Check sheet for the modelled part. Datum: model origin and axes. Units: mm. Face numbers are marked on the shaded views. A direction names the side the tool comes from. Coordinates: 2 decimals unless noted, no trailing zeros. Loops run counter-clockwise (first coordinate to the right, second up) from the corner with the lowest first, then second, coordinate; pieces in that order, holes last.
```python
from build123d import *
from build123d import SkipClean  # not in build123d's __all__

# Parameters (mm, degrees)
F0_R     = 37.5
F0_R_2   = 4.75
F1_DEPTH = 4
F2_DEPTH = 12


with BuildPart() as f1:
    # F0 (on Top) → F1 (new body)
    with BuildSketch(Plane.XY):
        Circle(F0_R)
        with BuildLine():
            ThreePointArc((3.5, 24.753787589), (18.8745860882, 16.3935963108), (25, 0))
            ThreePointArc((25, 0), (24.5426691937, -4.7599778204), (23.1874088919, -9.3458048812))
            ThreePointArc((23.1874088919, -9.3458048812), (21.6506350946, -12.5), (19.6874088919, -15.4079827077))
            ThreePointArc((19.6874088919, -15.4079827077), (0, -25), (-19.6874088919, -15.4079827077))
            ThreePointArc((-19.6874088919, -15.4079827077), (-21.6506350946, -12.5), (-23.1874088919, -9.3458048812))
            ThreePointArc((-23.1874088919, -9.3458048812), (-21.6506350946, 12.5), (-3.5, 24.753787589))
            ThreePointArc((-3.5, 24.753787589), (0, 25), (3.5, 24.753787589))
        make_face(mode=Mode.SUBTRACT)
        with BuildLine():
            Line((3.5, 21.719806629), (3.5, 24.753787589))
            ThreePointArc((3.5, 24.753787589), (0, 25), (-3.5, 24.753787589))
            Line((-3.5, 24.753787589), (-3.5, 21.719806629))
            ThreePointArc((-3.5, 21.719806629), (0, 22), (3.5, 21.719806629))
        make_face()
        with BuildLine():
            Line((3.5, 9.3674969976), (3.5, 21.719806629))
            ThreePointArc((3.5, 21.719806629), (0, 22), (-3.5, 21.719806629))
            Line((-3.5, 21.719806629), (-3.5, 9.3674969976))
            ThreePointArc((-3.5, 9.3674969976), (0, 10), (3.5, 9.3674969976))
        make_face()
        with BuildLine():
            ThreePointArc((17.059904306, -13.8909922277), (19.0525588833, -11), (20.559904306, -7.8288144012))
            Line((20.559904306, -7.8288144012), (9.8624903698, -1.6526595856))
            ThreePointArc((9.8624903698, -1.6526595856), (8.6602540378, -5), (6.3624903698, -7.714837412))
            Line((6.3624903698, -7.714837412), (17.059904306, -13.8909922277))
        make_face()
        with BuildLine():
            ThreePointArc((19.6874088919, -15.4079827077), (21.6506350946, -12.5), (23.1874088919, -9.3458048812))
            Line((23.1874088919, -9.3458048812), (20.559904306, -7.8288144012))
            ThreePointArc((20.559904306, -7.8288144012), (19.0525588833, -11), (17.059904306, -13.8909922277))
            Line((17.059904306, -13.8909922277), (19.6874088919, -15.4079827077))
        make_face()
        with BuildLine():
            Line((-9.8624903698, -1.6526595856), (-20.559904306, -7.8288144012))
            ThreePointArc((-20.559904306, -7.8288144012), (-19.0525588833, -11), (-17.059904306, -13.8909922277))
            Line((-17.059904306, -13.8909922277), (-6.3624903698, -7.714837412))
            ThreePointArc((-6.3624903698, -7.714837412), (-8.6602540378, -5), (-9.8624903698, -1.6526595856))
        make_face()
        with BuildLine():
            Line((-20.559904306, -7.8288144012), (-23.1874088919, -9.3458048812))
            ThreePointArc((-23.1874088919, -9.3458048812), (-21.6506350946, -12.5), (-19.6874088919, -15.4079827077))
            Line((-19.6874088919, -15.4079827077), (-17.059904306, -13.8909922277))
            ThreePointArc((-17.059904306, -13.8909922277), (-19.0525588833, -11), (-20.559904306, -7.8288144012))
        make_face()
        with BuildLine():
            ThreePointArc((10, 0), (8.2158383626, 5.7008771255), (3.5, 9.3674969976))
            ThreePointArc((3.5, 9.3674969976), (0, 10), (-3.5, 9.3674969976))
            ThreePointArc((-3.5, 9.3674969976), (-8.6602540378, 5), (-9.8624903698, -1.6526595856))
            ThreePointArc((-9.8624903698, -1.6526595856), (-8.6602540378, -5), (-6.3624903698, -7.714837412))
            ThreePointArc((-6.3624903698, -7.714837412), (0, -10), (6.3624903698, -7.714837412))
            ThreePointArc((6.3624903698, -7.714837412), (8.6602540378, -5), (9.8624903698, -1.6526595856))
            ThreePointArc((9.8624903698, -1.6526595856), (9.9655632981, -0.8291852332), (10, 0))
        make_face()
        Circle(F0_R_2, mode=Mode.SUBTRACT)
        with BuildLine():
            ThreePointArc((23.1874088919, -9.3458048812), (24.5426691937, -4.7599778204), (25, 0))
            ThreePointArc((25, 0), (18.8745860882, 16.3935963108), (3.5, 24.753787589))
            Line((3.5, 24.753787589), (3.5, 21.719806629))
            ThreePointArc((3.5, 21.719806629), (16.7481342244, 14.2653426177), (22, 0))
            ThreePointArc((22, 0), (21.6369810132, -3.9800819884), (20.559904306, -7.8288144012))
            Line((20.559904306, -7.8288144012), (23.1874088919, -9.3458048812))
        make_face()
        with BuildLine():
            ThreePointArc((-19.6874088919, -15.4079827077), (0, -25), (19.6874088919, -15.4079827077))
            Line((19.6874088919, -15.4079827077), (17.059904306, -13.8909922277))
            ThreePointArc((17.059904306, -13.8909922277), (0, -22), (-17.059904306, -13.8909922277))
            Line((-17.059904306, -13.8909922277), (-19.6874088919, -15.4079827077))
        make_face()
        with BuildLine():
            Line((-3.5, 21.719806629), (-3.5, 24.753787589))
            ThreePointArc((-3.5, 24.753787589), (-21.6506350946, 12.5), (-23.1874088919, -9.3458048812))
            Line((-23.1874088919, -9.3458048812), (-20.559904306, -7.8288144012))
            ThreePointArc((-20.559904306, -7.8288144012), (-19.0525588833, 11), (-3.5, 21.719806629))
        make_face()
    extrude(amount=F1_DEPTH)

    # F0 (on Top) → F2 (join)
    with BuildSketch(Plane.XY):
        with BuildLine():
            ThreePointArc((23.1874088919, -9.3458048812), (24.5426691937, -4.7599778204), (25, 0))
            ThreePointArc((25, 0), (18.8745860882, 16.3935963108), (3.5, 24.753787589))
            Line((3.5, 24.753787589), (3.5, 21.719806629))
            ThreePointArc((3.5, 21.719806629), (16.7481342244, 14.2653426177), (22, 0))
            ThreePointArc((22, 0), (21.6369810132, -3.9800819884), (20.559904306, -7.8288144012))
            Line((20.559904306, -7.8288144012), (23.1874088919, -9.3458048812))
        make_face()
        with BuildLine():
            Line((3.5, 21.719806629), (3.5, 24.753787589))
            ThreePointArc((3.5, 24.753787589), (0, 25), (-3.5, 24.753787589))
            Line((-3.5, 24.753787589), (-3.5, 21.719806629))
            ThreePointArc((-3.5, 21.719806629), (0, 22), (3.5, 21.719806629))
        make_face()
        with BuildLine():
            Line((-3.5, 21.719806629), (-3.5, 24.753787589))
            ThreePointArc((-3.5, 24.753787589), (-21.6506350946, 12.5), (-23.1874088919, -9.3458048812))
            Line((-23.1874088919, -9.3458048812), (-20.559904306, -7.8288144012))
            ThreePointArc((-20.559904306, -7.8288144012), (-19.0525588833, 11), (-3.5, 21.719806629))
        make_face()
        with BuildLine():
            Line((-20.559904306, -7.8288144012), (-23.1874088919, -9.3458048812))
            ThreePointArc((-23.1874088919, -9.3458048812), (-21.6506350946, -12.5), (-19.6874088919, -15.4079827077))
            Line((-19.6874088919, -15.4079827077), (-17.059904306, -13.8909922277))
            ThreePointArc((-17.059904306, -13.8909922277), (-19.0525588833, -11), (-20.559904306, -7.8288144012))
        make_face()
        with BuildLine():
            ThreePointArc((-19.6874088919, -15.4079827077), (0, -25), (19.6874088919, -15.4079827077))
            Line((19.6874088919, -15.4079827077), (17.059904306, -13.8909922277))
            ThreePointArc((17.059904306, -13.8909922277), (0, -22), (-17.059904306, -13.8909922277))
            Line((-17.059904306, -13.8909922277), (-19.6874088919, -15.4079827077))
        make_face()
        with BuildLine():
            ThreePointArc((19.6874088919, -15.4079827077), (21.6506350946, -12.5), (23.1874088919, -9.3458048812))
            Line((23.1874088919, -9.3458048812), (20.559904306, -7.8288144012))
            ThreePointArc((20.559904306, -7.8288144012), (19.0525588833, -11), (17.059904306, -13.8909922277))
            Line((17.059904306, -13.8909922277), (19.6874088919, -15.4079827077))
        make_face()
        with BuildLine():
            Line((3.5, 9.3674969976), (3.5, 21.719806629))
            ThreePointArc((3.5, 21.719806629), (0, 22), (-3.5, 21.719806629))
            Line((-3.5, 21.719806629), (-3.5, 9.3674969976))
            ThreePointArc((-3.5, 9.3674969976), (0, 10), (3.5, 9.3674969976))
        make_face()
        with BuildLine():
            ThreePointArc((17.059904306, -13.8909922277), (19.0525588833, -11), (20.559904306, -7.8288144012))
            Line((20.559904306, -7.8288144012), (9.8624903698, -1.6526595856))
            ThreePointArc((9.8624903698, -1.6526595856), (8.6602540378, -5), (6.3624903698, -7.714837412))
            Line((6.3624903698, -7.714837412), (17.059904306, -13.8909922277))
        make_face()
        with BuildLine():
            Line((-9.8624903698, -1.6526595856), (-20.559904306, -7.8288144012))
            ThreePointArc((-20.559904306, -7.8288144012), (-19.0525588833, -11), (-17.059904306, -13.8909922277))
            Line((-17.059904306, -13.8909922277), (-6.3624903698, -7.714837412))
            ThreePointArc((-6.3624903698, -7.714837412), (-8.6602540378, -5), (-9.8624903698, -1.6526595856))
        make_face()
        with BuildLine():
            ThreePointArc((10, 0), (8.2158383626, 5.7008771255), (3.5, 9.3674969976))
            ThreePointArc((3.5, 9.3674969976), (0, 10), (-3.5, 9.3674969976))
            ThreePointArc((-3.5, 9.3674969976), (-8.6602540378, 5), (-9.8624903698, -1.6526595856))
            ThreePointArc((-9.8624903698, -1.6526595856), (-8.6602540378, -5), (-6.3624903698, -7.714837412))
            ThreePointArc((-6.3624903698, -7.714837412), (0, -10), (6.3624903698, -7.714837412))
            ThreePointArc((6.3624903698, -7.714837412), (8.6602540378, -5), (9.8624903698, -1.6526595856))
            ThreePointArc((9.8624903698, -1.6526595856), (9.9655632981, -0.8291852332), (10, 0))
        make_face()
        Circle(F0_R_2, mode=Mode.SUBTRACT)
    with SkipClean():  # cleaning this boolean's faces spoils the solid; the shape is the same uncleaned
        extrude(amount=-F2_DEPTH)


solid = f1.part
```
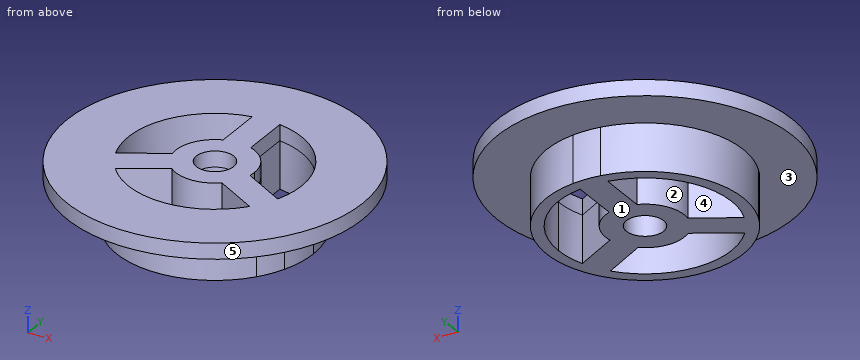
1) Depth check by flat-ended pin: pin 1 (1 mm diameter, centred on y = -14, z = -6, fed in from +X); pin 2 (11 mm diameter, centred on x = 0, y = 0, fed in from -Z); pin 3 (6 mm diameter, centred on x = -20, z = 2, fed in from +Y); pin 4 (3 mm diameter, centred on y = 17.5, z = 3, fed in from +X). Enter the tip coordinate at first touch or a pass-through.
Answer sheet:
pin 1: stops at x = 21.04
pin 2: stops at z = -12
pin 3: stops at y = 33.43
pin 4: stops at x = 33.92
2) Mould release check, pull along X, two halves, no side actions. Record for the marked faces 3, 4 and 5: +X half, -X half, draft (parallel to the pull), parting line (faces both ways), or undercut.
Answer sheet:
face 3: draft
face 4: undercut
face 5: parting line
3) Section check A-A on x = 0. Enter the section's corners in (y, z), plus the area to 3 significant figures.
Answer sheet:
outline: (-37.5, 0) - (-25, 0) - (-25, -12) - (-22, -12) - (-22, 4) - (-37.5, 4) - close; (-10, -12) - (-4.75, -12) - (-4.75, 4) - (-10, 4) - close; (4.75, -12) - (25, -12) - (25, 0) - (37.5, 0) - (37.5, 4) - (4.75, 4) - close
area: 556 mm2
4) Set-up check for the marked faces 1 and 2: record each of +Z, -Z, +X, -X, +Y, -Y from which the full face is reachable in a straight line by a thin tool's end or side.
Answer sheet:
face 1: -Z, +X, -X, +Y, -Y
face 2: +Z, -Z
5) Scan lines: line 1 (X direction, y = -2.5, z = -2); line 2 (X direction, y = -1.5, z = -11); line 3 (Y direction, x = -10.5, z = -3.5). Record each from-to range of solid material in increasing order.
Answer sheet:
line 1: x = -24.87 to -21.86, -11.33 to -4.04, 4.04 to 11.33, 21.86 to 24.87
line 2: x = -24.95 to -21.95, -9.89 to -4.51, 4.51 to 9.89, 21.95 to 24.95
line 3: y = -22.69 to -19.33, -10.1 to -2.02, 19.33 to 22.69
6) Section check C-C on z = -7. Enter the section's corners in (x, y), plus the area to 3 significant figures.
Answer sheet:
outline: circle Ø50 at (0, 0); hole (-20.56, -7.83) - (-9.86, -1.65) arc R10 cw to (-3.5, 9.37) - (-3.5, 21.72) arc R22 ccw to start; hole (-17.06, -13.89) arc R22 ccw to (17.06, -13.89) - (6.36, -7.71) arc R10 cw to (-6.36, -7.71) - close; hole circle Ø9.5 at (0, 0); hole (3.5, 9.37) arc R10 cw to (9.86, -1.65) - (20.56, -7.83) arc R22 ccw to (3.5, 21.72) - close
area: 941 mm2
7) Section check B-B on y = -17.5. Enter the section's corners in (x, z), plus the area to 3 significant figures.
Answer sheet:
outline: (-33.17, 0) - (-17.85, 0) - (-17.85, -12) - (-13.33, -12) - (-13.33, 4) - (-33.17, 4) - close; (13.33, -12) - (17.85, -12) - (17.85, 0) - (33.17, 0) - (33.17, 4) - (13.33, 4) - close
area: 267 mm2
8) Section check D-D on y = 13. Enter the section's corners in (x, z).
Answer sheet:
outline: (-35.17, 0) - (-21.35, 0) - (-21.35, -12) - (-17.75, -12) - (-17.75, 4) - (-35.17, 4) - close; (-3.5, -12) - (3.5, -12) - (3.5, 4) - (-3.5, 4) - close; (17.75, -12) - (21.35, -12) - (21.35, 0) - (35.17, 0) - (35.17, 4) - (17.75, 4) - close
